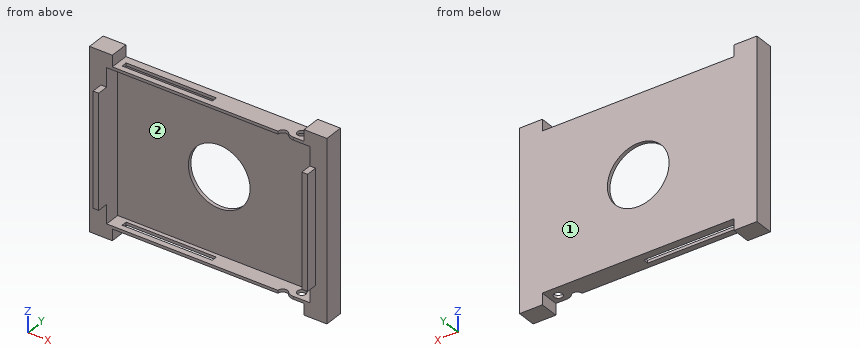
```python
from build123d import *

# Parameters (mm, degrees)
F0_R      = 16.25
F1_DEPTH  = 15.875
F2_W      = 139.2096877098
F2_H      = 115.5483946204
F2_W_2    = 113
F2_H_2    = 80
F3_DEPTH  = 5.875
F4_W      = 107
F4_H      = 80
F5_DEPTH  = 14
F6_W      = 120.5911301091
F6_H      = 13.1527084535
F6_W_2    = 121.3300417974
F6_H_2    = 15.8128053223
F7_DEPTH  = 5.875
F8_R      = 1.5
F8_W      = 89
F8_H      = 3
F9_DEPTH  = 100
F10_W     = 42.4407012761
F10_H     = 10
F11_DEPTH = 1.5
F12_W     = 42.5221920013
F12_H     = 10
F13_DEPTH = 1.5
F14_R     = 2.5
F15_DEPTH = 95.5
F16_R     = 2.25
F17_DEPTH = 200
F18_R     = 5


with BuildPart() as f1:
    # F0 (on Front) → F1 (new body)
    with BuildSketch(Plane.XZ):
        Polygon((-50.5, 47.5), (-62.5, 47.5), (-62.5, -47.5), (-50.5, -47.5), (-50.5, -41.5), (50.5, -41.5), (50.5, -47.5), (62.5, -47.5), (62.5, 47.5), (50.5, 47.5), (50.5, 41.5), (-50.5, 41.5), align=None)
        Circle(F0_R, mode=Mode.SUBTRACT)
    extrude(amount=F1_DEPTH)

    # F2 (on face) → F3 (cut)
    with BuildSketch(Plane.XZ.offset(15.875)):
        Rectangle(F2_W, F2_H)
        Rectangle(F2_W_2, F2_H_2, mode=Mode.SUBTRACT)
    extrude(amount=-F3_DEPTH, mode=Mode.SUBTRACT)

    # F4 (on face) → F5 (cut)
    with BuildSketch(Plane.XZ.offset(15.875)):
        Rectangle(F4_W, F4_H)
    extrude(amount=-F5_DEPTH, mode=Mode.SUBTRACT)

    # F6 (on face) → F7 (cut)
    with BuildSketch(Plane.XZ.offset(15.875)):
        with Locations((0.0607829645, 36.5763542267)):
            Rectangle(F6_W, F6_H)
        with Locations((1.0213727103, -37.9064026611)):
            Rectangle(F6_W_2, F6_H_2)
    extrude(amount=-F7_DEPTH, mode=Mode.SUBTRACT)

    # F8 (on face) → F9 (cut)
    with BuildSketch(Plane.XY.offset(41.5)):
        with Locations((46, -5.5)):
            Circle(F8_R)
        with Locations((-3, -5.5)):
            Rectangle(F8_W, F8_H)
    extrude(amount=-F9_DEPTH, mode=Mode.SUBTRACT)

    # F10 (on face) → F11 (join)
    with BuildSketch(Plane.XY.offset(41.5)):
        with Locations((21.220350638, -5)):
            Rectangle(F10_W, F10_H)
    extrude(amount=-F11_DEPTH)

    # F12 (on face) → F13 (join)
    with BuildSketch(Plane(origin=(0, 0, -41.5), x_dir=(1, 0, 0), z_dir=(0, 0, -1))):
        with Locations((21.2610960007, 5)):
            Rectangle(F12_W, F12_H)
    extrude(amount=-F13_DEPTH)

    # F14 (on face) → F15 (cut)
    with BuildSketch(Plane(origin=(0, 0, -41.5), x_dir=(1, 0, 0), z_dir=(0, 0, -1))):
        with Locations((39.25, 10)):
            Circle(F14_R)
    extrude(amount=-F15_DEPTH, mode=Mode.SUBTRACT)

    # F16 (on face) → F17 (cut)
    with BuildSketch(Plane.XY.offset(41.5)):
        with Locations((46, -5.5)):
            Circle(F16_R)
    extrude(amount=-F17_DEPTH, mode=Mode.SUBTRACT)

    # F18
    f18_edges = [f1.edges().sort_by_distance(p)[0] for p in [
        (41.75, -10, -40.75),
        (41.75, -10, 40.75),
    ]]
    fillet(f18_edges, radius=F18_R)


solid = f1.part
```
Here's how the part is built. I have some questions about the finished solid (model axes, mm). Face numbers are marked on the shaded views. A direction names the side the tool comes from. Coordinates: 2 decimals unless noted, no trailing zeros. Write each loop counter-clockwise with the first axis right and the second up, starting at its lowest first coordinate (ties: lowest second). Pieces come first, ordered by that corner, then holes. Notation, with made-up numbers: (0.25, 11.25) -> (58.25, 11.25) arc R21 cw to (58.25, 22.25) -> close; hole circle Ø10 at (-32.75, -11.5). An arc over 180 degrees is marked (long way). Use a Markdown table: item, result. Add a question column.
(1) If we section it at D-D, the plane x = 52: Write out the boundary of the cut face in (y, z) (3 decimals), and give its area (3 significant figures).
(2) Please list where these lines run through material, in increasing order: line 1 (X direction, y = -10.5, z = 11.5); line 2 (Z direction, x = 0, y = -0.9); line 3 (X direction, y = -8.5, z = -1.5).
(3) If we section it at C-C, the plane z = 0: Write out the boundary of the cut face in (x, y) (3 decimals), and give its area (3 significant figures).
(4) If we section it at A-A, the plane x = -35: Write out the boundary of the cut face in (y, z) (3 decimals).
(5) If we section it at B-B, the plane y = -5.5: State how many separate pieces and enclosed holes the cut face has, and give its area (3 significant figures).
(6) I'm going to push flat-ended pins straight in: P1, Ø0.9, axis at x = 54.5, y = -11.5, coming from the +Z side; P2, Ø4, axis at x = 21.5, y = -5.5, coming from the +Z side; P3, Ø2, axis at x = 43, z = 26.5, coming from the -Y side (3 decimals). Where does each tip first touch, or does it pass through?
(7) For the marked faces 1 and 2, which set-ups out of +Z, -Z, +X, -X, +Y, -Y let a thin tool reach every point of the face, with its end or its side?
Outcome:
| question | item | result |
|---|---|---|
| 1 | outline | (-10, -47.5) -> (0, -47.5) -> (0, 47.5) -> (-10, 47.5) -> (-10, 40) -> (-1.875, 40) -> (-1.875, -40) -> (-10, -40) -> close |
| 1 | area | 300 mm^2 |
| 2 | line 1 | x = -56.5 to -53.5, 53.5 to 56.5 |
| 2 | line 2 | z = -41.5 to -16.25, 16.25 to 41.5 |
| 2 | line 3 | x = -62.5 to -53.5, 53.5 to 62.5 |
| 3 | outline | (-62.5, -10) -> (-56.5, -10) -> (-56.5, -15.875) -> (-53.5, -15.875) -> (-53.5, -1.875) -> (-16.25, -1.875) -> (-16.25, 0) -> (-62.5, 0) -> close; (16.25, -1.875) -> (53.5, -1.875) -> (53.5, -15.875) -> (56.5, -15.875) -> (56.5, -10) -> (62.5, -10) -> (62.5, 0) -> (16.25, 0) -> close |
| 3 | area | 355 mm^2 |
| 4 | outline | (-10, -41.5) -> (-7, -41.5) -> (-7, -40) -> (-10, -40) -> close; (-10, 40) -> (-7, 40) -> (-7, 41.5) -> (-10, 41.5) -> close; (-4, -41.5) -> (0, -41.5) -> (0, 41.5) -> (-4, 41.5) -> (-4, 40) -> (-1.875, 40) -> (-1.875, -40) -> (-4, -40) -> close |
| 5 | separate pieces | 4 |
| 5 | enclosed holes | 0 |
| 5 | area | 1,950 mm^2 |
| 6 | P1 | stops at z = 30 |
| 6 | P2 | stops at z = 41.5 |
| 6 | P3 | stops at y = -1.875 |
| 7 | face 1 | +Z, -Z, +X, -X, +Y |
| 7 | face 2 | -Y |
